Geometry check sheet. Reference: the model listing, model coordinates, mm. Round coordinates to 2 decimals unless told otherwise and drop trailing zeros. Loops run counter-clockwise (first coordinate to the right, second up) from the corner with the lowest first, then second, coordinate; pieces in that order, holes last. Notation, with made-up numbers: (-14.5, 7.25) -> (9.5, 7.25) arc R18 ccw to (9.5, 36.25) -> close; hole circle Ø4 at (18, 29.25). An arc over 180 degrees is marked (long way). Use one line per item in the form item = value.
from build123d import *

# Parameters (mm, degrees)
F0_R     = 57.85
F0_R_2   = 17.5
F1_DEPTH = 15
F2_R     = 57.85
F2_R_2   = 55.35
F3_DEPTH = 3
F4_SIZE  = 5


with BuildPart() as f1:
    # F0 (on Front) → F1 (new body)
    with BuildSketch(Plane.XZ):
        Circle(F0_R)
        with BuildLine():
            ThreePointArc((-12.320414, -37.950196), (-10.329128, -41.855933), (-14.234864, -43.847219))
            ThreePointArc((-14.234864, -43.847219), (-23.05, -39.923771), (-30.855373, -34.251364))
            ThreePointArc((-30.855373, -34.251364), (-31.083737, -29.873254), (-26.705627, -29.64489))
            ThreePointArc((-26.705627, -29.64489), (-19.95, -34.554414), (-12.320414, -37.950196))
        make_face(mode=Mode.SUBTRACT)
        with BuildLine():
            ThreePointArc((-27.372431, 15.803481), (-25.159068, 13.141948), (-25.204864, 9.680642))
            ThreePointArc((-25.204864, 9.680642), (-27, 0), (-25.204864, -9.680642))
            ThreePointArc((-25.204864, -9.680642), (-25.159068, -13.141948), (-27.372431, -15.803481))
            Line((-27.372431, -15.803481), (-38.729833, -22.36068))
            ThreePointArc((-38.729833, -22.36068), (-42.790653, -22.780694), (-45.810926, -20.033948))
            ThreePointArc((-45.810926, -20.033948), (-50, 0), (-45.810926, 20.033948))
            ThreePointArc((-45.810926, 20.033948), (-42.790653, 22.780694), (-38.729833, 22.36068))
            Line((-38.729833, 22.36068), (-27.372431, 15.803481))
        make_face(mode=Mode.SUBTRACT)
        Circle(F0_R_2, mode=Mode.SUBTRACT)
        with BuildLine():
            Line((0, -44.72136), (0, -31.606961))
            ThreePointArc((0, -31.606961), (1.198273, -28.359366), (4.21875, -26.668374))
            ThreePointArc((4.21875, -26.668374), (13.5, -23.382686), (20.986114, -16.987731))
            ThreePointArc((20.986114, -16.987731), (23.960795, -15.217418), (27.372431, -15.803481))
            Line((27.372431, -15.803481), (38.729833, -22.36068))
            ThreePointArc((38.729833, -22.36068), (41.123986, -25.667445), (40.255371, -29.656452))
            ThreePointArc((40.255371, -29.656452), (25, -43.30127), (5.555556, -49.690399))
            ThreePointArc((5.555556, -49.690399), (1.666667, -48.44814), (0, -44.72136))
        make_face(mode=Mode.SUBTRACT)
        with BuildLine():
            ThreePointArc((45.090238, 9.595855), (46.1, 0), (45.090238, -9.595855))
            ThreePointArc((45.090238, -9.595855), (41.412865, -11.982679), (39.026041, -8.305306))
            ThreePointArc((39.026041, -8.305306), (39.9, 0), (39.026041, 8.305306))
            ThreePointArc((39.026041, 8.305306), (41.412865, 11.982679), (45.090238, 9.595855))
        make_face(mode=Mode.SUBTRACT)
        with BuildLine():
            ThreePointArc((-30.855373, 34.251364), (-23.05, 39.923771), (-14.234864, 43.847219))
            ThreePointArc((-14.234864, 43.847219), (-10.329128, 41.855933), (-12.320414, 37.950196))
            ThreePointArc((-12.320414, 37.950196), (-19.95, 34.554414), (-26.705627, 29.64489))
            ThreePointArc((-26.705627, 29.64489), (-31.083737, 29.873254), (-30.855373, 34.251364))
        make_face(mode=Mode.SUBTRACT)
        with BuildLine():
            ThreePointArc((20.986114, 16.987731), (13.5, 23.382686), (4.21875, 26.668374))
            ThreePointArc((4.21875, 26.668374), (1.198273, 28.359366), (0, 31.606961))
            Line((0, 31.606961), (0, 44.72136))
            ThreePointArc((0, 44.72136), (1.666667, 48.44814), (5.555556, 49.690399))
            ThreePointArc((5.555556, 49.690399), (25, 43.30127), (40.255371, 29.656452))
            ThreePointArc((40.255371, 29.656452), (41.123986, 25.667445), (38.729833, 22.36068))
            Line((38.729833, 22.36068), (27.372431, 15.803481))
            ThreePointArc((27.372431, 15.803481), (23.960795, 15.217418), (20.986114, 16.987731))
        make_face(mode=Mode.SUBTRACT)
    extrude(amount=F1_DEPTH)

    # F2 (on face) → F3 (cut)
    with BuildSketch(Plane(origin=(0, 0, 0), x_dir=(-1, 0, 0), z_dir=(0, 1, 0))):
        Circle(F2_R)
        Circle(F2_R_2, mode=Mode.SUBTRACT)
    extrude(amount=-F3_DEPTH, mode=Mode.SUBTRACT)

    # F4
    f4_edges = [f1.edges().sort_by_distance(p)[0] for p in [
        (-17.5, -15, 0),
    ]]
    chamfer(f4_edges, length=F4_SIZE)


solid = f1.part
1. Mould release check, pull along Z, two halves, no side actions. Record for faces 1 (the cylindrical face through (41.136, -7.395, 25.725)), 2 (the cylindrical face through (1.711, -7.395, -48.487)), 3 (the flat face through (-1, -15, -25)), 4 (the cylindrical face through (11.999, -1.479, -54.034)): released by +Z, released by -Z, zero draft, split by the parting line, or undercut.
Return value:
face_1 = undercut
face_2 = undercut
face_3 = zero draft
face_4 = split by the parting line
2. Section check B-B (x = -44). Record the boundary of the cut face in (y, z).
Return value:
outline = (-15, -37.56) -> (-3, -37.56) -> (-3, -33.58) -> (0, -33.58) -> (0, -22.19) -> (-15, -22.19) -> close; (-15, 22.19) -> (0, 22.19) -> (0, 33.58) -> (-3, 33.58) -> (-3, 37.56) -> (-15, 37.56) -> close
3. Section check A-A (z = 0). Record the boundary of the cut face in (x, y).
Return value:
outline = (-57.85, -15) -> (-50, -15) -> (-50, 0) -> (-55.35, 0) -> (-55.35, -3) -> (-57.85, -3) -> close; (-27, -15) -> (-22.5, -15) -> (-17.5, -10) -> (-17.5, 0) -> (-27, 0) -> close; (17.5, -10) -> (22.5, -15) -> (39.9, -15) -> (39.9, 0) -> (17.5, 0) -> close; (46.1, -15) -> (57.85, -15) -> (57.85, -3) -> (55.35, -3) -> (55.35, 0) -> (46.1, 0) -> close
4. Section check D-D (y = -5.75). Count the separate pieces of the cut face and the enclosed holes in it, then the cut area to 3 significant figures.
Return value:
separate_pieces = 1
enclosed_holes = 7
area = 6,410 mm2
5. Section check C-C (z = -47). Record the boundary of the cut face in (x, y).
Return value:
outline = (-33.73, -15) -> (0.55, -15) -> (0.55, 0) -> (-29.23, 0) -> (-29.23, -3) -> (-33.73, -3) -> close; (17.06, -15) -> (33.73, -15) -> (33.73, -3) -> (29.23, -3) -> (29.23, 0) -> (17.06, 0) -> close
6. Material ranges on line 1 along Z through (x, y) = (-11.5, -5.5); line 2 along X through (y, z) = (-13.5, 10.5); line 3 along X through (y, z) = (-5.75, 6.5), recorded low to high.
Return value:
line_1 = -56.7 to -43.44, -38.36 to -13.19, 13.19 to 38.36, 43.44 to 56.7
line_2 = -56.89 to -48.89, -24.97 to -18.19, 18.19 to 39.37, 44.74 to 56.89
line_3 = -57.48 to -49.58, -26.21 to -16.25, 16.25 to 39.37, 45.64 to 57.48
7. Gauge pin test, flat ends, axial feed: pin 1 (6 mm diameter, centred on x = 46, y = -11.5, fed in from +Z); pin 2 (1.5 mm diameter, centred on y = -6.5, z = 13, fed in from -X); pin 3 (2 mm diameter, centred on y = -3.5, z = -33.5, fed in from -X). Record the tip position at first contact, or that the pin passes through.
Return value:
pin_1 = 38.7
pin_2 = -56.54
pin_3 = -47.86
